Can you work these out from the model? Positions are in its coordinate system, mm. Face numbers are marked on the shaded views. A direction names the side the tool comes from. Round coordinates to 2 decimals unless told otherwise and drop trailing zeros. Loops run counter-clockwise (first coordinate to the right, second up) from the corner with the lowest first, then second, coordinate; pieces in that order, holes last.
(1) Thinking about a two-plate mould opening in X: for the marked faces 4, 5 and 6, which applies, released by +X, released by -X, zero draft, split by the parting line, or undercut?
(2) Will these pins go through, and if not, where does the flat tip stop? pin 1 Ø0.5 at (x, y) = (4, -1) entering from -Z; pin 2 Ø4 at (x, y) = (5.5, 5.5) entering from -Z; pin 3 Ø0.8 at (x, z) = (6.5, 0) entering from -Y.
(3) I want a section at A-A on z = -1.75. Write out the boundary of the cut face in (x, y).
(4) If I drill on line 1 along X through (y, z) = (2, -2); line 2 along Y through (x, z) = (4.75, -0.25); line 3 along Y through (x, z) = (2.5, -3.5), over which ranges is the centre line in solid material (lowest first)?
(5) I want a section at C-C on z = -5.5. Write out the boundary of the cut face in (x, y).
(6) Which directions (+Z, -Z, +X, -X, +Y, -Y) give clear straight access to the entire face, cutting with the end or side of a thin tool? Please do the marked faces 1, 2 and 3.
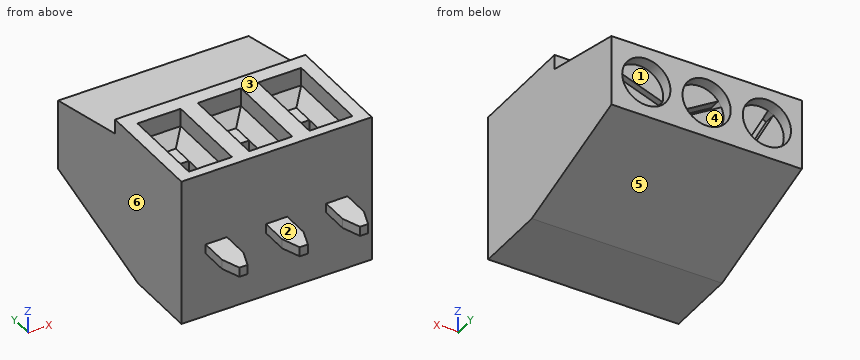
from build123d import *
from OCP.BRepFilletAPI import BRepFilletAPI_MakeChamfer
from build123d.topology import SkipClean

# Parameters (mm, degrees)
SKETCH1_W             = 8.02
SKETCH1_H             = 6.223
EXTRUDE1_DEPTH        = 8.636
CUT_EXTRUDE1_DEPTH    = 14.327663899
CUT_EXTRUDE2_DEPTH    = 14.327663899
SKETCH4_R             = 1.016
CUT_EXTRUDE3_DEPTH    = 0.508
SKETCH6_W             = 1.82195597
SKETCH6_H             = 3.601033201
CUT_EXTRUDE5_DEPTH    = 1.27
CHAMFER1_SIZE         = 0.508
CUT_EXTRUDE6_DEPTH    = 1.27
SKETCH8_W             = 0.9
SKETCH8_H             = 0.4
EXTRUDE2_DEPTH        = 1.905
CHAMFER2_SIZE         = 0.762
CHAMFER2_SIZE2        = 0.277345319
LPATTERN1_START       = 0.41494466
LPATTERN1_DEPTH       = 3.601033201
LPATTERN1_START_2     = 8.128
LPATTERN1_2_OUTLINE_R = 1.016
LPATTERN1_2_DEPTH     = 0.508
LPATTERN1_START_3     = 1.83446126
LPATTERN1_3_DEPTH     = 0.762
LPATTERN1_START_4     = -1.143
LPATTERN1_4_OUTLINE_W = 0.9
LPATTERN1_4_OUTLINE_H = 0.4
LPATTERN1_4_DEPTH     = 1.55794466
LPATTERN1_START_5     = -3.5
LPATTERN1_5_DEPTH     = 0.4
LPATTERN1_6_DEPTH     = 8
CUT_EXTRUDE4_START    = -0.508
CUT_EXTRUDE4_DEPTH    = 0.508


with BuildPart() as part:
    # Sketch1 → Extrude1 (new body)
    with BuildSketch(Plane(origin=(0, 0, 0), x_dir=(1, 0, 0), z_dir=(0, 1, 0))):
        with Locations((4.01, 3.1115)):
            Rectangle(SKETCH1_W, SKETCH1_H)
    extrude(amount=EXTRUDE1_DEPTH)

    # Sketch2 → Cut-Extrude1 (cut, through all)
    with BuildSketch(Plane(origin=(8.02, 0, 0), x_dir=(0, 0, -1), z_dir=(1, 0, 0))):
        Polygon((0, 4.645946632), (0.62179162, 4.645946632), (1.508470146, 8.636), (0, 8.636), align=None)
    extrude(amount=-CUT_EXTRUDE1_DEPTH, mode=Mode.SUBTRACT)

    # Sketch3 → Cut-Extrude2 (cut, through all)
    with BuildSketch(Plane(origin=(8.02, 0, 0), x_dir=(0, 0, -1), z_dir=(1, 0, 0))):
        Polygon((4.500853694, 8.636), (6.223, 3.053870593), (6.223, 8.636), align=None)
    extrude(amount=-CUT_EXTRUDE2_DEPTH, mode=Mode.SUBTRACT)

    # Sketch4 → Cut-Extrude3 (cut)
    with BuildSketch(Plane(origin=(0, 8.636, 0), x_dir=(1, 0, 0), z_dir=(0, 1, 0))):
        with Locations(Location((4.01, 3.00466192, 0), (0, 0, 270))):
            Circle(SKETCH4_R)
    extrude(amount=-CUT_EXTRUDE3_DEPTH, mode=Mode.SUBTRACT)

    # Sketch6 → Cut-Extrude5 (cut)
    with BuildSketch(Plane.XY):
        with Locations((4.01, 2.215461261)):
            Rectangle(SKETCH6_W, SKETCH6_H)
    extrude(amount=-CUT_EXTRUDE5_DEPTH, mode=Mode.SUBTRACT)

    # Chamfer1
    chamfer1_edges = [part.edges().sort_by_distance(p)[0] for p in [
        (4.01, 4.015977861, -1.27),
        (4.920977985, 2.21546126, -1.27),
        (4.01, 0.41494466, -1.27),
        (3.099022015, 2.21546126, -1.27),
    ]]
    chamfer(chamfer1_edges, length=CHAMFER1_SIZE)

    # Sketch7 → Cut-Extrude6 (cut)
    with BuildSketch(Plane.XY.offset(-1.27)):
        Polygon((3.607022015, 2.59646126), (3.607021944, 1.83446126), (4.412977985, 1.83446126), (4.412977985, 2.59646126), align=None)
    extrude(amount=-CUT_EXTRUDE6_DEPTH, mode=Mode.SUBTRACT)

    # Sketch8 → Extrude2 (add)
    with BuildSketch(Plane.XZ):
        with Locations((4.01, -3.3)):
            Rectangle(SKETCH8_W, SKETCH8_H)
    extrude(amount=EXTRUDE2_DEPTH)

    # Chamfer2: one chamfer whose edges measure the first distance from different faces: ONE call of the kernel's chamfer builder (chamfer() names one face for all edges)
    chamfer2_edges_1 = [part.edges().sort_by_distance(p)[0] for p in [
        (3.56, -1.905, -3.3),
    ]]
    chamfer2_side_1 = [part.faces().sort_by_distance(p)[0] for p in [
        (3.56, -0.9525, -3.3),
    ]]
    chamfer2_edges_2 = [part.edges().sort_by_distance(p)[0] for p in [
        (4.46, -1.905, -3.3),
    ]]
    chamfer2_side_2 = [part.faces().sort_by_distance(p)[0] for p in [
        (4.46, -0.9525, -3.3),
    ]]
    chamfer2 = BRepFilletAPI_MakeChamfer(part.part.solid().wrapped)
    for e in chamfer2_edges_1:
        chamfer2.Add(CHAMFER2_SIZE, CHAMFER2_SIZE2, e.wrapped, chamfer2_side_1[0].wrapped)  # the first distance lies on this face
    for e in chamfer2_edges_2:
        chamfer2.Add(CHAMFER2_SIZE, CHAMFER2_SIZE2, e.wrapped, chamfer2_side_2[0].wrapped)  # the first distance lies on this face
    add(Compound.cast(chamfer2.Shape()), mode=Mode.REPLACE)

    # LPattern1: read off the stored shape, not the designer's step
    # LPattern1 outline → LPattern1 (cut)
    with BuildSketch(Plane(origin=(0, 0, 0), x_dir=(1, 0, 0), z_dir=(0, 1, 0)).offset(LPATTERN1_START)):
        Polygon((7.460977985, 0.762), (6.952977985, 1.27), (6.147022015, 1.27), (5.639022015, 0.762), (5.639022015, 0), (7.460977985, 0), align=None)
        Polygon((0.559022015, 0), (2.380977985, 0), (2.380977985, 0.762), (1.872977985, 1.27), (1.067022015, 1.27), (0.559022015, 0.762), align=None)
    extrude(amount=LPATTERN1_DEPTH, mode=Mode.SUBTRACT)

    # LPattern1 2 outline → LPattern1 2 (cut)
    with BuildSketch(Plane(origin=(0, 0, 0), x_dir=(1, 0, 0), z_dir=(0, 1, 0)).offset(LPATTERN1_START_2)):
        with Locations((6.55, 3.00466192)):
            Circle(LPATTERN1_2_OUTLINE_R)
        with Locations((1.47, 3.00466192)):
            Circle(LPATTERN1_2_OUTLINE_R)
    extrude(amount=LPATTERN1_2_DEPTH, mode=Mode.SUBTRACT)

    # LPattern1 3 outline → LPattern1 3 (cut)
    with BuildSketch(Plane(origin=(0, 0, 0), x_dir=(1, 0, 0), z_dir=(0, 1, 0)).offset(LPATTERN1_START_3)):
        Polygon((6.147022015, 1.27), (6.952977985, 1.27), (6.952977985, 2.54), (6.147021944, 2.54), align=None)
        Polygon((1.067022015, 1.27), (1.872977985, 1.27), (1.872977985, 2.54), (1.067021944, 2.54), align=None)
    extrude(amount=LPATTERN1_3_DEPTH, mode=Mode.SUBTRACT)

    # LPattern1 4 outline → LPattern1 4 (add)
    with BuildSketch(Plane(origin=(0, 0, 0), x_dir=(1, 0, 0), z_dir=(0, 1, 0)).offset(LPATTERN1_START_4)):
        with Locations((1.47, 3.3)):
            Rectangle(LPATTERN1_4_OUTLINE_W, LPATTERN1_4_OUTLINE_H)
        with Locations((6.55, 3.3)):
            Rectangle(LPATTERN1_4_OUTLINE_W, LPATTERN1_4_OUTLINE_H)
    extrude(amount=LPATTERN1_4_DEPTH)

    # LPattern1 5 outline → LPattern1 5 (add)
    with BuildSketch(Plane.XY.offset(LPATTERN1_START_5)):
        Polygon((1.297345319, -1.905), (1.642654681, -1.905), (1.92, -1.143), (1.02, -1.143), align=None)
        Polygon((6.377345319, -1.905), (6.722654681, -1.905), (7, -1.143), (6.1, -1.143), align=None)
    extrude(amount=LPATTERN1_5_DEPTH)

    # LPattern1 6 outline → LPattern1 6 (add)
    with BuildSketch(Plane.YZ):
        Polygon((0.41494466, -1.27), (0.92294466, -1.27), (0.41494466, -0.762), align=None)
        Polygon((4.015977861, -1.27), (4.015977861, -0.762), (3.507977861, -1.27), align=None)
    extrude(amount=LPATTERN1_6_DEPTH)

    # Sketch5 → Cut-Extrude4 (cut)
    with SkipClean():  # the faces are left unmerged after this step: merging them gives an invalid solid
        with BuildSketch(Plane(origin=(0, 8.128, 0), x_dir=(1, 0, 0), z_dir=(0, 1, 0)).offset(CUT_EXTRUDE4_START)):
            with BuildLine():
                ThreePointArc((5.647513235, 3.471324151), (5.596258893, 3.354853153), (5.559965426, 3.232888875))
                Line((5.559965426, 3.232888875), (7.452486765, 2.537999689))
                ThreePointArc((7.452486765, 2.537999689), (7.503741107, 2.654470687), (7.540034574, 2.776434965))
                Line((7.540034574, 2.776434965), (5.647513235, 3.471324151))
            make_face()
            with BuildLine():
                ThreePointArc((3.08182296, 2.591450857), (3.140754275, 2.478669649), (3.213321028, 2.374139426))
                Line((3.213321028, 2.374139426), (4.93817704, 3.417872983))
                ThreePointArc((4.93817704, 3.417872983), (4.879245725, 3.530654191), (4.806678972, 3.635184414))
                Line((4.806678972, 3.635184414), (3.08182296, 2.591450857))
            make_face()
            with BuildLine():
                ThreePointArc((0.891932879, 2.169141481), (1.000906863, 2.103436294), (1.117239285, 2.051868197))
                Line((1.117239285, 2.051868197), (2.048067121, 3.840182359))
                ThreePointArc((2.048067121, 3.840182359), (1.939093137, 3.905887546), (1.822760715, 3.957455643))
                Line((1.822760715, 3.957455643), (0.891932879, 2.169141481))
            make_face()
        extrude(amount=CUT_EXTRUDE4_DEPTH, mode=Mode.SUBTRACT)


solid = part.part
Filled sheet:
1. face 4: undercut
1. face 5: zero draft
1. face 6: released by -X
2. pin 1: stops at z = -3.5
2. pin 2: stops at z = -6.09
2. pin 3: stops at y = 0
3. outline: (0, 0) - (8.02, 0) - (8.02, 8.64) - (0, 8.64) - close; hole (1.07, 1.83) - (1.87, 1.83) - (1.87, 2.6) - (1.07, 2.6) - close; hole (3.61, 1.83) - (4.41, 1.83) - (4.41, 2.6) - (3.61, 2.6) - close; hole (6.15, 1.83) - (6.95, 1.83) - (6.95, 2.6) - (6.15, 2.6) - close
4. line 1: x = 0 to 1.07, 1.87 to 3.61, 4.41 to 6.15, 6.95 to 8.02
4. line 2: y = 0 to 0.41, 4.02 to 4.65
4. line 3: y = 0 to 8.64
5. outline: (0, 0) - (8.02, 0) - (8.02, 5.4) - (0, 5.4) - close
6. face 1: +Y
6. face 2: +Z, +X, -X, -Y
6. face 3: +Z, +X, -X, +Y, -Y
